from build123d import *

# Parameters (mm, degrees)
SKETCH1_R               = 4
BOSS_EXTRUDE1_DEPTH     = 3
SKETCH2_R               = 6.5
BOSS_EXTRUDE2_DEPTH     = 102
SKETCH3_R               = 3.5
CUT_EXTRUDE1_DEPTH      = 110.230261375
CUT_EXTRUDE2_DEPTH      = 64.806347647
CUT_EXTRUDE2_DEPTH_BACK = 64.806347647
SKETCH4_W               = 53
SKETCH4_H               = 14.5
FILLET1_R               = 1.5
CHAMFER1_SIZE           = 1


with BuildPart() as part:
    # Sketch1 → Boss-Extrude1 (new body)
    with BuildSketch(Plane.XY):
        with BuildLine():
            Line((-51, 0), (51, 0))
            Line((51, 0), (51, 27.5))
            ThreePointArc((51, 27.5), (48.071067812, 34.571067812), (41, 37.5))
            Line((41, 37.5), (-41, 37.5))
            ThreePointArc((-41, 37.5), (-48.071067812, 34.571067812), (-51, 27.5))
            Line((-51, 27.5), (-51, 0))
        make_face()
        with Locations((-38, 18.5)):
            Circle(SKETCH1_R, mode=Mode.SUBTRACT)
        with Locations((38, 18.5)):
            Circle(SKETCH1_R, mode=Mode.SUBTRACT)
        with Locations((-12.5, 27.5)):
            Circle(SKETCH1_R, mode=Mode.SUBTRACT)
        with Locations((12.5, 27.5)):
            Circle(SKETCH1_R, mode=Mode.SUBTRACT)
    extrude(amount=BOSS_EXTRUDE1_DEPTH)

    # Sketch2 → Boss-Extrude2 (add)
    with BuildSketch(Plane.ZY.offset(51)):
        with Locations((4.5, 0)):
            Circle(SKETCH2_R)
    extrude(amount=-BOSS_EXTRUDE2_DEPTH)

    # Sketch3 → Cut-Extrude1 (cut, through all)
    with BuildSketch(Plane.ZY.offset(51)):
        with Locations((4.5, 0)):
            Circle(SKETCH3_R)
    extrude(amount=-CUT_EXTRUDE1_DEPTH, mode=Mode.SUBTRACT)

    # Sketch4 → Cut-Extrude2 (cut, two sides: drawn at the far end of the back side and taken through both)
    with BuildSketch(Plane.XY.offset(3).offset(-CUT_EXTRUDE2_DEPTH_BACK)):
        with Locations((0, 0.75)):
            Rectangle(SKETCH4_W, SKETCH4_H)
    extrude(amount=CUT_EXTRUDE2_DEPTH + CUT_EXTRUDE2_DEPTH_BACK, mode=Mode.SUBTRACT)

    # Fillet1
    fillet1_edges = [part.edges().sort_by_distance(p)[0] for p in [
        (-26.5, 8, 1.5),
        (26.5, 8, 1.5),
    ]]
    fillet(fillet1_edges, radius=FILLET1_R)

    # Chamfer1
    chamfer1_edges = [part.edges().sort_by_distance(p)[0] for p in [
        (-42, 18.5, 3),
        (34, 18.5, 3),
        (-16.5, 27.5, 3),
        (8.5, 27.5, 3),
    ]]
    chamfer(chamfer1_edges, length=CHAMFER1_SIZE)


solid = part.part
Can you work these out from the model? Positions are in its coordinate system, mm. A direction names the side the tool comes from. Coordinates: 2 decimals unless noted, no trailing zeros. Order: outer loops, then holes, each group sorted by start corner. A loop starts at its lowest first (then second) coordinate and runs counter-clockwise, first axis right, second up. Notation, with made-up numbers: M 30,13 L 35,13 A24 ccw 35,45 Z; hole C -11.75,-17 d7. An arc over 180 degrees is marked long. Write item = value, one per line.
(1) Suppose I cut it at A-A on x = 38. Please give me the cut outline in (y, z).
Results are:
outline = M 4.69,0 L 14.5,0 L 14.5,2 L 13.5,3 L 6.32,3 A6.5 ccw long Z; M 22.5,0 L 37.5,0 L 37.5,3 L 23.5,3 L 22.5,2 Z; hole C 0,4.5 d7
(2) Suppose I cut it at C-C on x = 12.5. Please give me the cut outline in (y, z), plus the area to 3 significant figures.
Results are:
outline = M 8,0 L 23.5,0 L 23.5,2 L 22.5,3 L 8,3 Z; M 31.5,0 L 37.5,0 L 37.5,3 L 32.5,3 L 31.5,2 Z
area = 63.5 mm2
(3) If we mould it in two halves opening along X, with no side actions, what happens to faces 3 (the face through (11.979, 31.466, 0.986)), 4 (the face through (48.15, 34.49, 1.48)), 5 (the face through (-39, -6, 7)), 6 (the face through (26.5, 3, 7))? For each: pulls with the +X half, pulls with the -X half, needs draft (parallel to the pull), parting line crosses it, or undercut.
Results are:
face_3 = undercut
face_4 = pulls with the +X half
face_5 = needs draft
face_6 = undercut
(4) For faces 1 (the face through (0, 8, 1)), 2 (the face through (-40.95, 21.2, 0.99)), which set-ups out of +Z, -Z, +X, -X, +Y, -Y let a thin tool reach every point of the face, with its end or its side?
Results are:
face_1 = +Z, -Z, -Y
face_2 = +Z, -Z
(5) For pin 1 Ø5 at (x, y) = (30, -1.5) entering from -Z; pin 2 Ø2 at (x, y) = (5.5, 25.5) entering from -Z; pin 3 Ø6 at (y, z) = (31, 2.5) entering from +X; pin 4 Ø3.5 at (x, z) = (9, 2) entering from -Y, each with a flat end and sliding along its axis, tell me the tip position at first contact or that it passes through.
Results are:
pin_1 = -2
pin_2 = 0
pin_3 = 50.99
pin_4 = 8
(6) I need wall thicknesses on line 1 along Y through (x, z) = (34.75, 4.5); line 2 along Y through (x, z) = (-38, 1.45); line 3 along Z through (x, y) = (45, 23.5). Which ranges of each line are inside material? Lowest first, please. Write a range as [from, to].
Results are:
line_1 = [-6.5, -3.5], [3.5, 6.5]
line_2 = [-5.74, -1.72], [1.72, 14.5], [22.5, 37.5]
line_3 = [0, 3]
(7) Suppose I cut it at B-B on y = 0. Please give me the cut outline in (x, z), plus the area to 3 significant figures.
Results are:
outline = M -51,-2 L -26.5,-2 L -26.5,1 L -51,1 Z; M -51,8 L -26.5,8 L -26.5,11 L -51,11 Z; M 26.5,-2 L 51,-2 L 51,1 L 26.5,1 Z; M 26.5,8 L 51,8 L 51,11 L 26.5,11 Z
area = 294 mm2
(8) Suppose I cut it at D-D on y = 17.5. State how many separate pieces and enclosed holes the cut face has, plus the area to 3 significant figures.
Results are:
separate_pieces = 3
enclosed_holes = 0
area = 257 mm2
